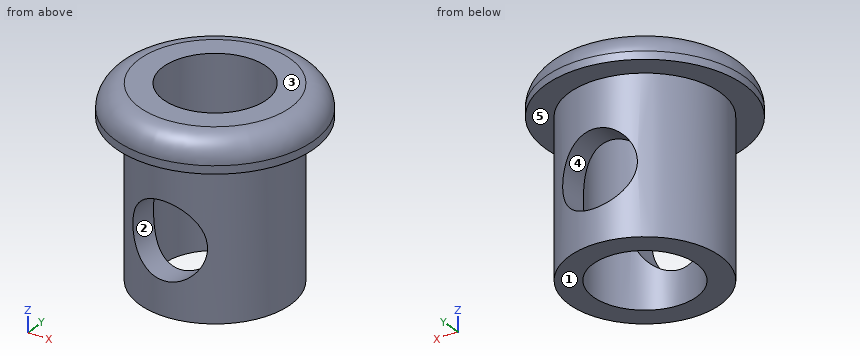
```python
from build123d import *

# Parameters (mm, degrees)
F0_R          = 9.5
F0_R_2        = 6.5
F1_DEPTH      = 19.5
F2_R          = 12.5
F2_R_2        = 6.5
F3_DEPTH      = 4
F4_R          = 3
F5_R          = 4.75
F6_DEPTH      = 25
F6_DEPTH_BACK = 25


with BuildPart() as f1:
    # F0 (on Top) → F1 (new body)
    with BuildSketch(Plane.XY):
        Circle(F0_R)
        Circle(F0_R_2, mode=Mode.SUBTRACT)
    extrude(amount=F1_DEPTH)

    # F2 (on face) → F3 (join)
    with BuildSketch(Plane.XY.offset(19.5)):
        Circle(F2_R)
        Circle(F2_R_2, mode=Mode.SUBTRACT)
    extrude(amount=F3_DEPTH)

    # F4
    f4_edges = [f1.edges().sort_by_distance(p)[0] for p in [
        (-12.5, 0, 23.5),
    ]]
    fillet(f4_edges, radius=F4_R)

    # F5 (on Front) → F6 (cut, two sides)
    with BuildSketch(Plane.XZ) as f6_sk:
        with Locations((0, 9)):
            Circle(F5_R)
    extrude(amount=-F6_DEPTH, mode=Mode.SUBTRACT)
    extrude(f6_sk.sketch, amount=F6_DEPTH_BACK, mode=Mode.SUBTRACT)


solid = f1.part
```
Geometry: final body of the model. Coordinates: model frame, mm. Face numbers are marked on the shaded views. A direction names the side the tool comes from. Coordinates: 2 decimals unless noted, no trailing zeros. Order: outer loops, then holes, each group sorted by start corner. A loop starts at its lowest first (then second) coordinate and runs counter-clockwise, first axis right, second up. Notation, with made-up numbers: M 33.5,10 L 73.5,10 A18 ccw 73.5,31 Z; hole C 42,32 d10. An arc over 180 degrees is marked long. Answer as CSV lines item,"result".
Q1. Section C-C on z = 11. Return the cut outline in (x, y), and give its area (3 significant figures).
Answers:
outline,"M -4.31,-8.47 L -4.31,-4.87 A6.5 cw -4.31,4.87 L -4.31,8.47 A9.5 ccw Z; M 4.31,-8.47 A9.5 ccw 4.31,8.47 L 4.31,4.87 A6.5 cw 4.31,-4.87 Z"
area,"96.0 mm^2"
Q2. Line query: probe 1 along Y at (x, z) = (0.25, 19.25); probe 2 along Z at (x, y) = (0, 6.95); probe 3 along Z at (x, y) = (-7, 6.75). Output: solid intervals per line, ascending. Write a range as [from, to].
Answers:
probe 1,"y = [-9.5, -6.5], [6.5, 9.5]"
probe 2,"z = [0, 4.25], [13.75, 23.5]"
probe 3,"z = [19.5, 23.49]"
Q3. Section D-D on z = 18. Return the cut outline in (x, y), and give its area (3 significant figures).
Answers:
outline,"C 0,0 d19; hole C 0,0 d13"
area,"151 mm^2"
Q4. Section A-A on x = 0. Return the cut outline in (y, z).
Answers:
outline,"M -12.5,19.5 L -9.5,19.5 L -9.5,13.75 L -6.5,13.75 L -6.5,23.5 L -9.5,23.5 A3 ccw -12.5,20.5 Z; M -9.5,0 L -6.5,0 L -6.5,4.25 L -9.5,4.25 Z; M 6.5,0 L 9.5,0 L 9.5,4.25 L 6.5,4.25 Z; M 6.5,13.75 L 9.5,13.75 L 9.5,19.5 L 12.5,19.5 L 12.5,20.5 A3 ccw 9.5,23.5 L 6.5,23.5 Z"
Q5. Set-up query: the marked faces 4 and 5. Return all of +Z, -Z, +X, -X, +Y, -Y with unobstructed straight access to the full face (end or side cutting, diameter ignored); none if empty.
Answers:
face 4,"+Y, -Y"
face 5,"-Z"
Q6. Draft query along Z for the marked faces 1, 2 and 3. Return one class per face: pulls with the +Z half, pulls with the -Z half, needs draft (parallel to the pull), parting line crosses it, or undercut.
Answers:
face 1,"pulls with the -Z half"
face 2,"undercut"
face 3,"pulls with the +Z half"
Q7. First-contact query: P1, Ø7.5, axis at x = 0, z = 9, coming from the -Y side; P2, Ø2, axis at x = 9, z = 3.5, coming from the -Y side; P3, Ø4, axis at x = 8, z = 12, coming from the -Y side; P4, Ø5, axis at y = -2, z = 16.5, coming from the +X side. Flat tips, straight axial feed; report the tip coordinate or a pass-through.
Answers:
P1,"passes through"
P2,"stops at y = -5.12"
P3,"stops at y = -7.37"
P4,"stops at x = 9.5"
Q8. Section B-B on y = 0. Return the cut outline in (x, z).
Answers:
outline,"M -12.5,19.5 L -9.5,19.5 L -9.5,0 L -6.5,0 L -6.5,23.5 L -9.5,23.5 A3 ccw -12.5,20.5 Z; M 6.5,0 L 9.5,0 L 9.5,19.5 L 12.5,19.5 L 12.5,20.5 A3 ccw 9.5,23.5 L 6.5,23.5 Z"
